```python
from build123d import *

# Parameters (mm, degrees)
F0_W      = 25
F0_H      = 25
F1_DEPTH  = 10
F5_W      = 22
F5_H      = 7
F6_DEPTH  = 25
F7_W      = 22
F7_H      = 7
F8_DEPTH  = 25
F9_W      = 20
F9_H      = 20
F10_DEPTH = 5
F11_W     = 2.5
F11_H     = 2.5
F12_DEPTH = 3
F3_W      = 20
F3_H      = 3
F13_DEPTH = 5


with BuildPart() as f1:
    # F0 (on Top) → F1 (new body)
    with BuildSketch(Plane.XY):
        Rectangle(F0_W, F0_H)
    extrude(amount=F1_DEPTH)

    # F5 (on face) → F6 (cut)
    with BuildSketch(Plane.XZ.offset(12.5)):
        with Locations((0, 5)):
            Rectangle(F5_W, F5_H)
    extrude(amount=-F6_DEPTH, mode=Mode.SUBTRACT)

    # F7 (on face) → F8 (cut)
    with BuildSketch(Plane.YZ.offset(12.5)):
        with Locations((0, 5)):
            Rectangle(F7_W, F7_H)
    extrude(amount=-F8_DEPTH, mode=Mode.SUBTRACT)

    # F9 (on face) → F10 (cut)
    with BuildSketch(Plane(origin=(0, 0, 0), x_dir=(1, 0, 0), z_dir=(0, 0, -1))):
        Rectangle(F9_W, F9_H)
    extrude(amount=-F10_DEPTH, mode=Mode.SUBTRACT)

    # F11 (on face) → F12 (join)
    with BuildSketch(Plane(origin=(0, 0, 0), x_dir=(1, 0, 0), z_dir=(0, 0, -1))):
        with Locations((11.25, 11.25)):
            Rectangle(F11_W, F11_H)
        with Locations((-11.25, 11.25)):
            Rectangle(F11_W, F11_H)
        with Locations((-11.25, -11.25)):
            Rectangle(F11_W, F11_H)
        with Locations((11.25, -11.25)):
            Rectangle(F11_W, F11_H)
    extrude(amount=F12_DEPTH)

    # F3 (on face) → F13 (cut)
    with BuildSketch(Plane.XY.offset(10)):
        with Locations((0, -8.75)):
            Rectangle(F3_W, F3_H)
        with Locations((0, 8.75)):
            Rectangle(F3_W, F3_H)
    extrude(amount=-F13_DEPTH, mode=Mode.SUBTRACT)


solid = f1.part
```
Could you check a few things on this model? Use its own coordinates, in mm. A direction names the side the tool comes from. Round coordinates to 2 decimals unless told otherwise and drop trailing zeros. Loops run counter-clockwise (first coordinate to the right, second up) from the corner with the lowest first, then second, coordinate; pieces in that order, holes last.
Q1. Thinking about a two-plate mould opening in Z: for faces 6 (the flat face through (-11, 0, 1.5)), 7 (the flat face through (-11, 0, 0)), 8 (the flat face through (-10, 0, 1)), which applies, pulls with the +Z half, pulls with the -Z half, needs draft (parallel to the pull), parting line crosses it, or undercut?
Q2. I want a section at A-A (z = 4.5). Write out the boundary of the cut face in (x, y).
Q3. I want a section at C-C (y = 5.75). Write out the boundary of the cut face in (x, z), and give its area (3 significant figures).
Q4. I want a section at B-B (x = 4). Write out the boundary of the cut face in (y, z), and give its area (3 significant figures).
Q5. For P1, Ø3, axis at x = -4.5, z = 6.5, coming from the +Y side; P2, Ø3, axis at x = 11, y = 3.5, coming from the -Z side, each with a flat end and sliding along its axis, tell me the tip position at first contact or that it passes through.
Q6. I want a section at D-D (y = 9). Write out the boundary of the cut face in (x, z).
Q7. On a 3-axis mill with a long thin cutter (end or side, diameter ignored), from which of +Z, -Z, +X, -X, +Y, -Y can I reach the whole of each face in a straight line? I mean faces 1 (the flat face through (10, 0, 1)), 2 (the flat face through (0, 11, 0)), 3 (the flat face through (-12, -11, 5)), 4 (the flat face through (11, 0, 0)), 5 (the flat face through (0, 0, 10)). Say none if no direction works.
Q8. Please list where these lines run through material, in increasing order: L1, parallel to Z at x = -11, y = -2.75; L2, parallel to X at y = 11.5, z = 8; L3, parallel to Z at x = 4, y = -5.
Answer below:
1. face 6: undercut
1. face 7: pulls with the -Z half
1. face 8: needs draft
2. outline: (-12.5, -12.5) - (-11, -12.5) - (-11, -11) - (-12.5, -11) - close; (-12.5, 11) - (-11, 11) - (-11, 12.5) - (-12.5, 12.5) - close; (11, -12.5) - (12.5, -12.5) - (12.5, -11) - (11, -11) - close; (11, 11) - (12.5, 11) - (12.5, 12.5) - (11, 12.5) - close
3. outline: (-12.5, 0) - (-10, 0) - (-10, 1.5) - (-12.5, 1.5) - close; (-12.5, 8.5) - (12.5, 8.5) - (12.5, 10) - (-12.5, 10) - close; (10, 0) - (12.5, 0) - (12.5, 1.5) - (10, 1.5) - close
3. area: 45.0 mm2
4. outline: (-12.5, 0) - (-10, 0) - (-10, 1.5) - (-12.5, 1.5) - close; (-12.5, 8.5) - (-10.25, 8.5) - (-10.25, 10) - (-12.5, 10) - close; (-7.25, 8.5) - (7.25, 8.5) - (7.25, 10) - (-7.25, 10) - close; (10, 0) - (12.5, 0) - (12.5, 1.5) - (10, 1.5) - close; (10.25, 8.5) - (12.5, 8.5) - (12.5, 10) - (10.25, 10) - close
4. area: 36.0 mm2
5. P1: passes through
5. P2: stops at z = 0
6. outline: (-12.5, 0) - (-10, 0) - (-10, 1.5) - (-12.5, 1.5) - close; (-12.5, 8.5) - (-10, 8.5) - (-10, 10) - (-12.5, 10) - close; (10, 0) - (12.5, 0) - (12.5, 1.5) - (10, 1.5) - close; (10, 8.5) - (12.5, 8.5) - (12.5, 10) - (10, 10) - close
7. face 1: -Z
7. face 2: -Z, +Y, -Y
7. face 3: +X, -X
7. face 4: -Z, +X, -X
7. face 5: +Z, +X, -X, +Y, -Y
8. L1: z = 0 to 1.5, 8.5 to 10
8. L2: x = -12.5 to -11, 11 to 12.5
8. L3: z = 8.5 to 10
